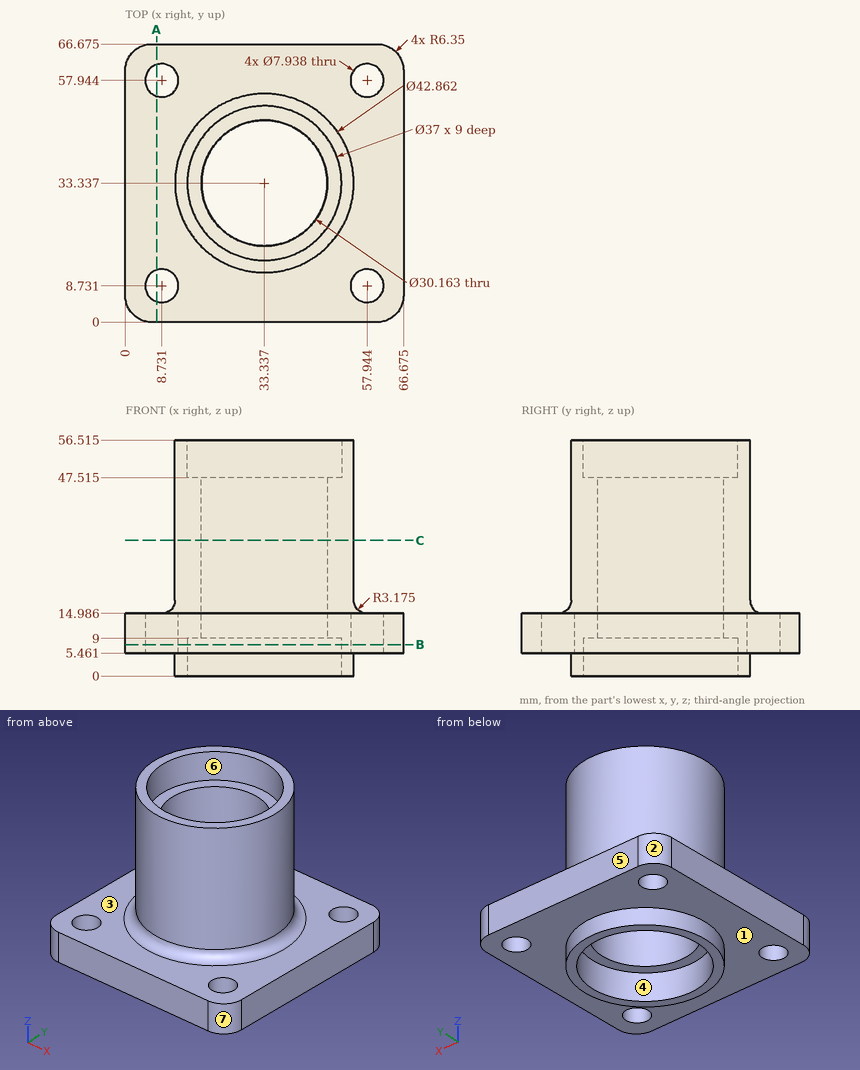
Geometry: see drawing. Coordinates: mm, zero at the bounding-box minimum. A direction names the side the tool comes from. Coordinates: 2 decimals unless noted, no trailing zeros. Loops run counter-clockwise (first coordinate to the right, second up) from the corner with the lowest first, then second, coordinate; pieces in that order, holes last. Notation, with made-up numbers: (16.5, 26.25) -> (20.5, 26.25) arc R13 cw to (20.5, 46.25) -> close; hole circle Ø9 at (21, 13.5). An arc over 180 degrees is marked (long way). Use a Markdown table: item, result.
1) Access query for the marked faces 1, 2 and 3. Directions: +Z, -Z, +X, -X, +Y, -Y. A direction counts if a zero-diameter tool reaches every point of the face in a straight line with its end or side. Return the directions, or none.
Results found:
| item | result |
|---|---|
| face 1 | -Z |
| face 2 | +Z, -Z, -X, +Y |
| face 3 | +Z |
2) Material intervals for line 1 along Y through (x, z) = (31, 35.5) (1 decimal); line 2 along Z through (x, y) = (45, 22) (1 decimal); line 3 along Y through (x, z) = (26, 50.5) (1 decimal), sorted ascending. Write a range as from..to.
Results found:
| item | result |
|---|---|
| line 1 | y = 12..18.4, 48.2..54.6 |
| line 2 | z = 9..47.5 |
| line 3 | y = 13.2..16.4, 50.3..53.5 |
3) Cut plane C-C (z = 32.5). Return the cut outline in (x, y).
Results found:
| item | result |
|---|---|
| outline | circle Ø42.86 at (33.34, 33.34); hole circle Ø30.16 at (33.34, 33.34) |
4) Contact query for flat-ended pins moving along their axis: pin 1 (1 mm diameter, centred on x = 50.5, y = 38.5, fed in from -Z); pin 2 (6 mm diameter, centred on x = 15, z = 19, fed in from -Y); pin 3 (1.5 mm diameter, centred on x = 28.5, z = 49.5, fed in from +Y) (1 decimal). Output: stop coordinate, or through.
Results found:
| item | result |
|---|---|
| pin 1 | stops at z = 9 |
| pin 2 | stops at y = 18.37 |
| pin 3 | stops at y = 54.4 |
5) Cut plane A-A (x = 7.5). Return the cut outline in (y, z) (1 decimal).
Results found:
| item | result |
|---|---|
| outline | (0, 5.5) -> (5, 5.5) -> (5, 15) -> (0, 15) -> close; (12.5, 5.5) -> (54.2, 5.5) -> (54.2, 15) -> (12.5, 15) -> close; (61.7, 5.5) -> (66.7, 5.5) -> (66.7, 15) -> (61.7, 15) -> close |
6) Cut plane B-B (z = 7.5). Give the number of separate pieces and of enclosed holes in the cut face, then the cut area to 3 significant figures.
Results found:
| item | result |
|---|---|
| separate pieces | 1 |
| enclosed holes | 5 |
| area | 3,140 mm2 |
7) Pull-direction query (X, two-part tool) for the marked faces 4, 5, 6 and 7; classes: released by +X, released by -X, zero draft, split by the parting line, or undercut.
Results found:
| item | result |
|---|---|
| face 4 | undercut |
| face 5 | zero draft |
| face 6 | undercut |
| face 7 | released by +X |
